```python
from build123d import *

# Parameters (mm, degrees)
F1_DEPTH  = 16
F2_W      = 70
F2_H      = 3
F3_DEPTH  = 2
F4_W      = 50
F4_H      = 14
F5_DEPTH  = 2
F6_R      = 0.99999
F9_DEPTH  = 2
F11_DEPTH = 38.001
F13_D     = 4
F14_R     = 3
F14_R_2   = 2
F15_DEPTH = 5
F16_R     = 3


# Not quite as in the source:
# - a fillet or chamfer is up to 0.001 mm smaller than in the source, because OpenCascade refuses the exact size
# - a pattern or mirror of a feature is missing from the dataset's text; its kind, count and spacing are read off the source's solid


with BuildPart() as f1:
    # F0 (on Front) → F1 (new body)
    with BuildSketch(Plane.XZ):
        with BuildLine():
            Line((94, 9), (0, 9))
            ThreePointArc((0, 9), (-9, 0), (0, -9))
            Line((0, -9), (19, -9))
            ThreePointArc((19, -9), (21.9107246536, -9.9345748081), (23.7333333333, -12.3889272035))
            ThreePointArc((23.7333333333, -12.3889272035), (40.3930033582, -39.2216179023), (67.1516242057, -56))
            ThreePointArc((67.1516242057, -56), (72.9993471235, -57.3376618382), (77.7503977132, -61))
            Line((77.7503977132, -61), (79.1305544342, -59.4934290732))
            ThreePointArc((79.1305544342, -59.4934290732), (73.8943105869, -55.5314515361), (67.507653226, -54.0062881394))
            ThreePointArc((67.507653226, -54.0062881394), (41.6996239436, -37.699069728), (25.6266664621, -11.7444981545))
            ThreePointArc((25.6266664621, -11.7444981545), (23.0750143892, -8.308404907), (19, -7.0000002161))
            Line((19, -7.0000002161), (0, -7.0000002161))
            ThreePointArc((0, -7.0000002161), (-7.0000002161, 0), (0, 7.0000002161))
            Line((0, 7.0000002161), (94, 7.0000002161))
            Line((94, 7.0000002161), (94, 9))
        make_face()
    extrude(amount=F1_DEPTH)

    # F2 (on face) → F3 (join)
    with BuildSketch(Plane.XY.offset(9)):
        with Locations((59, -17.5)):
            Rectangle(F2_W, F2_H)
    extrude(amount=-F3_DEPTH)

    # F4 (on face) → F5 (join)
    with BuildSketch(Plane.XZ.offset(19)):
        with Locations((69, 2)):
            Rectangle(F4_W, F4_H)
    extrude(amount=-F5_DEPTH)

    # F6 (radius 1 in the source; OpenCascade refuses exactly that, so slightly less here)
    f6_edges = [f1.edges().sort_by_distance(p)[0] for p in [
        (69, -17, 7),
        (59, -19, 9),
    ]]
    fillet(f6_edges, radius=F6_R)

    # F7: F1 across face


with BuildPart() as f1_1:
    add(f1.part)
    add(f1.part.mirror(Plane(origin=(37.3146952464, 0, -11.3167767816), x_dir=(1, 0, 0), z_dir=(0, 1, 0))))

    # F8 (on face) → F9 (cut)
    with BuildSketch(Plane.XY.offset(9)):
        with BuildLine():
            Line((94, 11.9899458001), (34.491120871, 11.9899458001))
            ThreePointArc((34.491120871, 11.9899458001), (22.0000006537, 0.0039610115), (34.4832053788, -11.9902674099))
            Line((34.4832053788, -11.9902674099), (94, -11.9902674099))
            Line((94, -11.9902674099), (94, 11.9899458001))
        make_face()
    extrude(amount=-F9_DEPTH, mode=Mode.SUBTRACT)

    # F10 (on face) → F11 (cut, through all)
    with BuildSketch(Plane.XZ.offset(19)):
        with BuildLine():
            ThreePointArc((50, 3), (47, 0), (50, -3))
            Line((50, -3), (70, -3))
            ThreePointArc((70, -3), (73, 0), (70, 3))
            Line((70, 3), (50, 3))
        make_face()
    extrude(amount=-F11_DEPTH, mode=Mode.SUBTRACT)

    # F13 (through all)
    with Locations(Plane.XZ.offset(19)):
        with Locations((80, 1)):
            Hole(F13_D / 2)

    # F14 (on face) → F15 (join)
    with BuildSketch(Plane(origin=(0, -17, 0), x_dir=(-1, 0, 0), z_dir=(0, 1, 0))):
        with Locations((-80, 1)):
            Circle(F14_R)
        with Locations((-80, 1)):
            Circle(F14_R_2, mode=Mode.SUBTRACT)
    f15 = extrude(amount=F15_DEPTH)

    # F15_copies: F15 across plane
    add(f15.mirror(Plane.ZX))

    # F16
    f16_edges = [f1_1.edges().sort_by_distance(p)[0] for p in [
        (94, 18, -5),
        (94, -18, -5),
        (44, -18, -5),
        (44, 18, -5),
    ]]
    fillet(f16_edges, radius=F16_R)


solid = f1_1.part
```
The model under review builds one solid part; all positions refer to its coordinate system, in mm. A direction names the side the tool comes from. Round coordinates to 2 decimals unless told otherwise and drop trailing zeros. Loops run counter-clockwise (first coordinate to the right, second up) from the corner with the lowest first, then second, coordinate; pieces in that order, holes last. Notation, with made-up numbers: (-26.5, 67.5) -> (-11.5, 67.5) arc R17 cw to (-11.5, 80.5) -> close; hole circle Ø10 at (-4, -19). An arc over 180 degrees is marked (long way). Answer as a JSON object with one key per item and string values. Group by question number.
1) Mouldability with a two-part tool opening along Z and no side actions: class faces 4 (the face through (69, 18, -5)), 5 (the face through (60, -18, -3)), 6 (the face through (94, -18, 5)) as released by +Z, released by -Z, zero draft, split by the parting line, or undercut.
2) We need section D-D on z = 1. Give the number of separate pieces and of enclosed holes in the cut face, then the cut area to 3 significant figures.
3) For pin 1 Ø5 at (x, z) = (80, 1) entering from -Y; pin 2 Ø2 at (x, y) = (79, 18.5) entering from -Z; pin 3 Ø1.5 at (y, z) = (-17.5, 1) entering from -X; pin 4 Ø5 at (x, y) = (7, -1) entering from -Z, all flat-tipped, find the tip position at first contact; note any pin that passes through.
4) We need section A-A on x = 32.5. Write out the cut boundary in (y, z).
5) We need section C-C on y = 8. Write out the cut boundary in (x, z).
6) For faces 1 (the face through (60, -18, 3)), 2 (the face through (79, -12, -1)), 3 (the face through (44, 18, 2)), list the 3-axis set-ups (+Z, -Z, +X, -X, +Y, -Y) from which the entire face can be reached by the end or side of a thin tool; tool diameter is ignored.
7) For line 1 (Z direction, x = 80, y = 14.75); line 2 (Z direction, x = 80, y = -18); line 3 (Z direction, x = 11.5, y = -7.5), list the stretches that pass through material, from the lowest coordinate up. Write a range as [from, to].
8) We need section B-B on x = 59. Write out the cut boundary in (y, z), then the cut area to 3 significant figures.
Result set:
{
 "1": {"face 4": "released by -Z", "face 5": "undercut", "face 6": "zero draft"},
 "2": {"separate pieces": "7", "enclosed holes": "0", "area": "166 mm²"},
 "3": {"pin 1": "y = -19", "pin 2": "z = -5", "pin 3": "x = 44", "pin 4": "z = -9"},
 "4": {"outline": "(-19, 7) -> (-11.91, 7) -> (-11.91, 9) -> (-18, 9) arc R1 ccw to (-19, 8) -> close; (-16, -29.76) -> (16, -29.76) -> (16, -26.13) -> (-16, -26.13) -> close; (11.91, 7) -> (19, 7) -> (19, 8) arc R1 ccw to (18, 9) -> (11.91, 9) -> close"},
 "5": {"outline": "(0, -9) -> (19, -9) arc R5 cw to (23.73, -12.39) arc R70 ccw to (67.15, -56) arc R14 cw to (77.75, -61) -> (79.13, -59.49) arc R16 ccw to (67.51, -54.01) arc R68 cw to (25.63, -11.74) arc R7 ccw to (19, -7) -> (0, -7) arc R7 cw to (0, 7) -> (25.06, 7) -> (25.06, 9) -> (0, 9) arc R9 ccw to start"},
 "6": {"face 1": "+Y, -Y", "face 2": "+Z, +X", "face 3": "-Z, -X, +Y, -Y"},
 "7": {"line 1": "[-2, -1], [3, 4], [7, 9]", "line 2": "[-5, -1], [3, 9]", "line 3": "[-9, -7], [7, 9]"},
 "8": {"outline": "(-19, -5) -> (-17, -5) -> (-17, -3) -> (-19, -3) -> close; (-19, 3) -> (-17, 3) -> (-17, 6) arc R1 cw to (-16, 7) -> (-11.99, 7) -> (-11.99, 9) -> (-18, 9) arc R1 ccw to (-19, 8) -> close; (-16, -52.6) -> (16, -52.6) -> (16, -50.36) -> (-16, -50.36) -> close; (11.99, 7) -> (16, 7) arc R1 cw to (17, 6) -> (17, 3) -> (19, 3) -> (19, 8) arc R1 ccw to (18, 9) -> (11.99, 9) -> close; (17, -5) -> (19, -5) -> (19, -3) -> (17, -3) -> close", "area": "124 mm²"}
}
